Geometry check sheet. Reference: the model listing, model coordinates, mm. A direction names the side the tool comes from. Round coordinates to 2 decimals unless told otherwise and drop trailing zeros. Loops run counter-clockwise (first coordinate to the right, second up) from the corner with the lowest first, then second, coordinate; pieces in that order, holes last. Notation, with made-up numbers: M 82.5,78 L 106.5,78 A23 cw 106.5,103 Z; hole C 59.5,-24.5 d6. An arc over 180 degrees is marked long. Use one line per item in the form item = value. Start each with the question number.
1. Material ranges on line 1 (Z direction, x = -5.75, y = -2); line 2 (X direction, y = 1.75, z = 56); line 3 (X direction, y = -2, z = 78.5), recorded low to high.
2. Go/stop test with flat-tipped pins: pin 1 (1 mm diameter, centred on x = -6.5, z = 30.5, fed in from -Y); pin 2 (1.5 mm diameter, centred on x = -6, y = -2, fed in from -Z); pin 3 (1.5 mm diameter, centred on x = 2.5, z = 16, fed in from -Y). Record where each tip stops, or that it passes through.
3. Draft check along Z on faces 1 (the flat face through (6, 0, 34)), 2 (the cylindrical face through (-4.824, 12.014, 77.486)), 3 (the flat face through (6, -1, 2)), 4 (the flat face through (5.25, 5, 43)). Enter one of: pulls with the +Z half, pulls with the -Z half, needs draft (parallel to the pull), parting line crosses it, or undercut.
4. Set-up check for faces 5 (the flat face through (5.35, -1, 44)), 6 (the flat face through (-6, -3, 7)), 7 (the cylindrical face through (-4.824, 12.014, 37.486)), 8 (the flat face through (6, -1, 12)), 9 (the flat face through (0.6, 11.3, 0)): record each of +Z, -Z, +X, -X, +Y, -Y from which the full face is reachable in a straight line by a thin tool's end or side.
5. Cross-section at C-C (x = 0.5). State how many separate pieces and enclosed holes the cut face has, then the cut area to 3 significant figures.
6. Cross-section at B-B (z = 41.5). Record the boundary of the cut face in (x, y), then the cut area to 3 significant figures.
7. Cross-section at A-A (y = 0.75). Record the boundary of the cut face in (x, z).
```python
from build123d import *

# Parameters (mm, degrees)
EXTRUDE_1_DEPTH     = 88
CUT_EXTRUDE_1_DEPTH = 55
SKETCH_4_W          = 1.9
SKETCH_4_H          = 10
EXTRUDE_2_DEPTH     = 3


with BuildPart() as part:
    # 草图1 → 凸台-拉伸1 (new body)
    with BuildSketch(Plane.XY):
        Polygon((-7.25, 0), (-7.25, 13), (7.25, 13), (7.25, 0), (5.25, 0), (5.25, 11), (-5.25, 11), (-5.25, 0), align=None)
    extrude(amount=EXTRUDE_1_DEPTH)

    # 草图2 → 切除-拉伸1 (cut)
    with BuildSketch(Plane(origin=(0, 13, 0), x_dir=(1, 0, 0), z_dir=(0, 1, 0))):
        with BuildLine():
            Line((-3, -5.621760717), (3, -5.621760717))
            ThreePointArc((3, -5.621760717), (4.824580314, -7.44634103), (3, -9.270921344))
            Line((3, -9.270921344), (-3, -9.270921344))
            ThreePointArc((-3, -9.270921344), (-4.824580314, -7.44634103), (-3, -5.621760717))
        make_face()
        with BuildLine():
            Line((-3, -15.621760717), (3, -15.621760717))
            ThreePointArc((3, -15.621760717), (4.824580314, -17.44634103), (3, -19.270921344))
            Line((3, -19.270921344), (-3, -19.270921344))
            ThreePointArc((-3, -19.270921344), (-4.824580314, -17.44634103), (-3, -15.621760717))
        make_face()
        with BuildLine():
            Line((-3, -25.621760717), (3, -25.621760717))
            ThreePointArc((3, -25.621760717), (4.824580314, -27.44634103), (3, -29.270921344))
            Line((3, -29.270921344), (-3, -29.270921344))
            ThreePointArc((-3, -29.270921344), (-4.824580314, -27.44634103), (-3, -25.621760717))
        make_face()
        with BuildLine():
            Line((-3, -35.621760717), (3, -35.621760717))
            ThreePointArc((3, -35.621760717), (4.824580314, -37.44634103), (3, -39.270921344))
            Line((3, -39.270921344), (-3, -39.270921344))
            ThreePointArc((-3, -39.270921344), (-4.824580314, -37.44634103), (-3, -35.621760717))
        make_face()
        with BuildLine():
            Line((-3, -45.621760717), (3, -45.621760717))
            ThreePointArc((3, -45.621760717), (4.824580314, -47.44634103), (3, -49.270921344))
            Line((3, -49.270921344), (-3, -49.270921344))
            ThreePointArc((-3, -49.270921344), (-4.824580314, -47.44634103), (-3, -45.621760717))
        make_face()
        with BuildLine():
            Line((-3, -55.621760717), (3, -55.621760717))
            ThreePointArc((3, -55.621760717), (4.824580314, -57.44634103), (3, -59.270921344))
            Line((3, -59.270921344), (-3, -59.270921344))
            ThreePointArc((-3, -59.270921344), (-4.824580314, -57.44634103), (-3, -55.621760717))
        make_face()
        with BuildLine():
            Line((-3, -65.621760717), (3, -65.621760717))
            ThreePointArc((3, -65.621760717), (4.824580314, -67.44634103), (3, -69.270921344))
            Line((3, -69.270921344), (-3, -69.270921344))
            ThreePointArc((-3, -69.270921344), (-4.824580314, -67.44634103), (-3, -65.621760717))
        make_face()
        with BuildLine():
            Line((-3, -75.621760717), (3, -75.621760717))
            ThreePointArc((3, -75.621760717), (4.824580314, -77.44634103), (3, -79.270921344))
            Line((3, -79.270921344), (-3, -79.270921344))
            ThreePointArc((-3, -79.270921344), (-4.824580314, -77.44634103), (-3, -75.621760717))
        make_face()
    extrude(amount=-CUT_EXTRUDE_1_DEPTH, mode=Mode.SUBTRACT)

    # 草图4 → 凸台-拉伸2 (add)
    with BuildSketch(Plane.XZ):
        with Locations((6.3, 80)):
            Rectangle(SKETCH_4_W, SKETCH_4_H)
        with Locations((6.3, 44)):
            Rectangle(SKETCH_4_W, SKETCH_4_H)
        with Locations((6.3, 7)):
            Rectangle(SKETCH_4_W, SKETCH_4_H)
    extrude_2 = extrude(amount=EXTRUDE_2_DEPTH)

    # 镜向1: 凸台-拉伸2 across plane
    add(extrude_2.mirror(Plane(origin=(0, 0, 0), x_dir=(0, 0, 1), z_dir=(1, 0, 0))))


solid = part.part
```
Reported:
q1.line_1 = 2 to 12, 39 to 49, 75 to 85
q1.line_2 = -7.25 to -5.25, 5.25 to 7.25
q1.line_3 = -7.25 to -5.35, 5.35 to 7.25
q2.pin_1 = 0
q2.pin_2 = 2
q2.pin_3 = 11
q3.face_1 = undercut
q3.face_2 = undercut
q3.face_3 = pulls with the -Z half
q3.face_4 = needs draft
q4.face_5 = +Z, -Z, -Y
q4.face_6 = +Z, -Z, +X, -X, -Y
q4.face_7 = +Y, -Y
q4.face_8 = +X, -X, -Y
q4.face_9 = -Z, +X, -X, +Y, -Y
q5.separate_pieces = 9
q5.enclosed_holes = 0
q5.area = 118 mm²
q6.outline = M -7.25,-3 L -5.35,-3 L -5.35,0 L -5.25,0 L -5.25,11 L 5.25,11 L 5.25,0 L 5.35,0 L 5.35,-3 L 7.25,-3 L 7.25,13 L -7.25,13 Z
q6.area = 84.4 mm²
q7.outline = M -7.25,0 L -5.25,0 L -5.25,88 L -7.25,88 Z; M 5.25,0 L 7.25,0 L 7.25,88 L 5.25,88 Z
